Verification items for this drawing (mm, ordinates from the low corner). A direction names the side the tool comes from. Coordinates: 2 decimals unless noted, no trailing zeros. Order: outer loops, then holes, each group sorted by start corner. A loop starts at its lowest first (then second) coordinate and runs counter-clockwise, first axis right, second up.
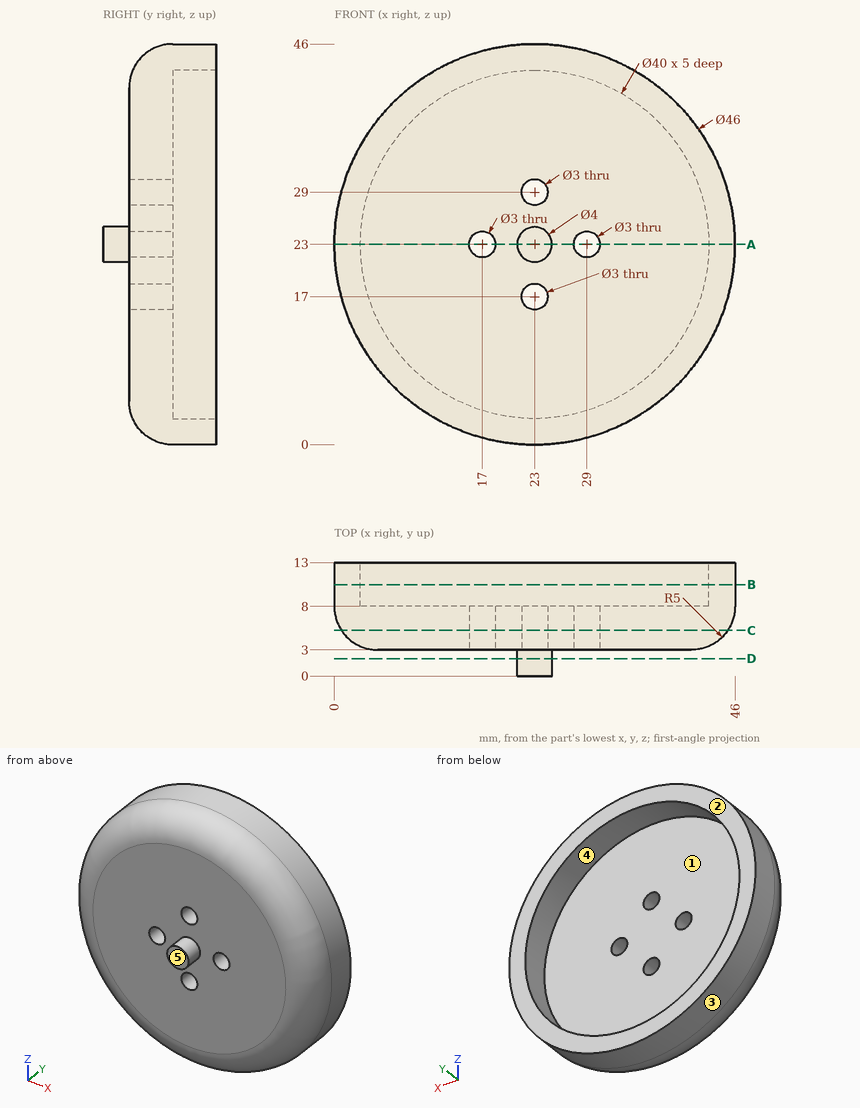
(1) Tool access check on the marked faces 1 and 2. Record the directions out of +Z, -Z, +X, -X, +Y, -Y that give a thin tool (end or side, any length) a straight path to the whole face; none if there is none.
Filled in:
face 1: +Y
face 2: +Z, -Z, +X, -X, +Y
(2) Cross-section at B-B (y = 10.5). Enter the section's corners in (x, z).
Filled in:
outline: circle Ø46 at (23, 23); hole circle Ø40 at (23, 23)
(3) Cross-section at A-A (z = 23). Enter the section's corners in (x, y).
Filled in:
outline: (0, 8) arc R5 ccw to (5, 3) - (15.5, 3) - (15.5, 8) - (3, 8) - (3, 13) - (0, 13) - close; (18.5, 3) - (21, 3) - (21, 0) - (25, 0) - (25, 3) - (27.5, 3) - (27.5, 8) - (18.5, 8) - close; (30.5, 3) - (41, 3) arc R5 ccw to (46, 8) - (46, 13) - (43, 13) - (43, 8) - (30.5, 8) - close
(4) Thickness scan on probe 1 along X at (y, z) = (5.6, 23); probe 2 along Y at (x, z) = (21, 10); probe 3 along X at (y, z) = (8.75, 38). Record the ranges inside material, lowest first.
Filled in:
probe 1: x = 0.61 to 15.5, 18.5 to 27.5, 30.5 to 45.39
probe 2: y = 3 to 8
probe 3: x = 5.56 to 9.77, 36.23 to 40.44
(5) Cross-section at C-C (y = 5.25). Enter the section's corners in (x, z).
Filled in:
outline: circle Ø44.35 at (23, 23); hole circle Ø3 at (17, 23); hole circle Ø3 at (23, 17); hole circle Ø3 at (23, 29); hole circle Ø3 at (29, 23)
(6) Release check for a two-part mould opening along X. For the marked faces 3, 4 and 5 record: +X half, -X half, draft (parallel to the pull), parting line (faces both ways), or undercut.
Filled in:
face 3: parting line
face 4: undercut
face 5: draft
(7) Go/stop test with flat-tipped pins: P1, Ø2, axis at y = 4, z = 12.5, coming from the -X side; P2, Ø10, axis at x = 6.5, z = 6, coming from the -Y side; P3, Ø2, axis at y = 8.5, z = 37.5, coming from the -X side; P4, Ø3, axis at x = 20.5, z = 24.5, coming from the -Y side. Record where each tip stops, or that it passes through.
Filled in:
P1: stops at x = 3.52
P2: stops at y = 3.05
P3: stops at x = 4.38
P4: stops at y = 0
(8) Cross-section at D-D (y = 2). Enter the section's corners in (x, z).
Filled in:
outline: circle Ø4 at (23, 23)
